```python
from build123d import *

# Parameters (mm, degrees)
F3_DEPTH = 25.4
F5_DEPTH = 30.481
F6_SIZE  = 2.54


with BuildPart() as f1:
    # F0 (on Top) → F1 (revolve)
    with BuildSketch(Plane.XY):
        Polygon((-9.8806, 0), (-7.3406, 0), (-7.3406, 15.24), (-18.288, 15.24), (-18.288, 21.59), (-6.096, 21.59), (-6.096, 24.13), (-17.272, 24.13), (-17.272, 33.02), (-6.096, 33.02), (-6.096, 38.1), (-17.272, 38.1), (-20.32, 35.56), (-20.32, 12.7), (-9.8806, 12.7), align=None)
    revolve(axis=Axis((0, 12.155764, 0), (0, 1, 0)))

    # F2 (on face) → F3 (cut)
    with BuildSketch(Plane(origin=(0, 38.1, 0), x_dir=(-1, 0, 0), z_dir=(0, 1, 0))):
        with BuildLine():
            Line((-15.24, -13.440417), (-15.24, 13.440417))
            ThreePointArc((-15.24, 13.440417), (-20.32, 0), (-15.24, -13.440417))
        make_face()
        with BuildLine():
            ThreePointArc((15.24, -13.440417), (20.32, 0), (15.24, 13.440417))
            Line((15.24, 13.440417), (15.24, -13.440417))
        make_face()
    extrude(amount=-F3_DEPTH, mode=Mode.SUBTRACT)

    # F4 (on face) → F5 (cut, through all)
    with BuildSketch(Plane.YZ.offset(15.24)):
        Polygon((12.7, 25.189353), (12.7, 18.839353), (38.1, 13.440417), (38.1, 25.189353), align=None)
    extrude(amount=-F5_DEPTH, mode=Mode.SUBTRACT)

    # F6
    f6_edges = [f1.edges().sort_by_distance(p)[0] for p in [
        (9.8806, 12.7, 0),
    ]]
    chamfer(f6_edges, length=F6_SIZE)


solid = f1.part
```
Part model, mm, in its own coordinate system. A direction names the side the tool comes from. Round coordinates to 2 decimals unless told otherwise and drop trailing zeros. Write each loop counter-clockwise with the first axis right and the second up, starting at its lowest first coordinate (ties: lowest second). Pieces come first, ordered by that corner, then holes. Notation, with made-up numbers: M 73,8.25 L 89,8.25 A31 ccw 89,33.25 Z; hole C 49,3 d9. An arc over 180 degrees is marked long. One line per question, with ' | ' between items.
(1) 3-axis set-ups, long thin cutter, end or side, ignore diameter. For faces 4 (the face through (-12.26, 28.637, 12.166)), 5 (the face through (13.948, 37.377, 11.598)), 6 (the face through (0, 12.7, 13)): which of +Z, -Z, +X, -X, +Y, -Y reach the whole face in a straight line?
Answer key:
face 4: none | face 5: +Z, +X, +Y | face 6: -Y
(2) Saw through at A-A on z = 0. Count the separate pieces of the cut face and the enclosed holes in it, then the cut area to 3 significant figures.
Answer key:
separate pieces: 6 | enclosed holes: 0 | area: 250 mm^2
(3) Saw through at C-C on y = 29.5. Write the cut outline in (x, z).
Answer key:
outline: M -15.24,-13.44 A20.32 ccw 15.24,-13.44 L 15.24,-8.13 A17.27 cw -15.24,-8.13 Z; M -15.24,8.13 A17.27 cw -8.07,15.27 L -13.41,15.27 A20.32 ccw -15.24,13.44 Z; M 8.07,15.27 A17.27 cw 15.24,8.13 L 15.24,13.44 A20.32 ccw 13.41,15.27 Z
(4) Probe line 1 along Y through (x, z) = (11.5, 6); line 2 along Y through (x, z) = (7.5, -3.5); line 3 along Z through (x, y) = (0, 3.5). List the from-to ranges inside material, lowest first.
Answer key:
line 1: y = 12.7 to 15.24, 21.59 to 24.13, 33.02 to 38.1 | line 2: y = 0 to 15.24, 21.59 to 24.13, 33.02 to 38.1 | line 3: z = -9.88 to -7.34, 7.34 to 9.88
(5) Pin check, flat tips, straight feed: pin 1 (4 mm diameter, centred on y = 9, z = 9, fed in from -X); pin 2 (12 mm diameter, centred on x = -7.5, y = 9, fed in from +Z); pin 3 (3 mm diameter, centred on x = -9.5, y = 10, fed in from +Z); pin 4 (4 mm diameter, centred on x = 9.5, y = 21.5, fed in from -Z). Stop position of each tip, or through.
Answer key:
pin 1: stops at x = -6.97 | pin 2: stops at z = 18.84 | pin 3: stops at z = 6.73 | pin 4: stops at z = -18.89
(6) Two-plate mould, pull along X, no slides. Class faces 1 (the face through (-4.6, 10.3, -8.9)), 2 (the face through (7, 24.13, 0)), 3 (the face through (0.206, 22.4, 16.778)): released by +X, released by -X, zero draft, split by the parting line, or undercut.
Answer key:
face 1: split by the parting line | face 2: undercut | face 3: zero draft
(7) Saw through at D-D on y = 5. Write the cut outline in (x, z).
Answer key:
outline: C 0,0 d19.76; hole C 0,0 d14.68
